from build123d import *

# Parameters (mm, degrees)
SKETCH1_R                             = 7.9375
BOSS_EXTRUDE1_DEPTH                   = 53.467
F_29_0_136_DIAMETER_HOLE1_D           = 3.4544
F_29_0_136_DIAMETER_HOLE1_CSINK_D     = 4.7244
F_29_0_136_DIAMETER_HOLE1_CSINK_ANGLE = 45
F_15_0_18_DIAMETER_HOLE1_D            = 4.572
F_53_0_0595_DIAMETER_HOLE1_D          = 1.5113
F_3_8_0_375_DIAMETER_HOLE1_D          = 9.525
F_3_8_0_375_DIAMETER_HOLE1_DEPTH      = 50.8
F_3_8_0_375_DIAMETER_HOLE1_TIP        = 2.861598698
F_39_0_0995_DIAMETER_HOLE1_D          = 2.54


with BuildPart() as part:
    # Sketch1 → Boss-Extrude1 (new body)
    with BuildSketch(Plane(origin=(0, 0, 0), x_dir=(1, 0, 0), z_dir=(0, 1, 0))):
        with Locations(Location((0, 0, 0), (0, 0, 270))):
            Circle(SKETCH1_R)
    extrude(amount=BOSS_EXTRUDE1_DEPTH)

    # #29 (0.136) Diameter Hole1 (through all)
    with Locations(Plane.XY.offset(7.9375)):
        with Locations((0, 49.022)):
            CounterSinkHole(F_29_0_136_DIAMETER_HOLE1_D / 2, F_29_0_136_DIAMETER_HOLE1_CSINK_D / 2, counter_sink_angle=F_29_0_136_DIAMETER_HOLE1_CSINK_ANGLE)

    # #15 (0.18) Diameter Hole1 (through all)
    with Locations(Plane.XY.offset(7.9375)):
        with Locations((0, 40.64)):
            Hole(F_15_0_18_DIAMETER_HOLE1_D / 2)

    # #53 (0.0595) Diameter Hole1 (through all)
    with Locations(Plane.XY.offset(7.9375)):
        with Locations((0, 32.639)):
            Hole(F_53_0_0595_DIAMETER_HOLE1_D / 2)

    # 3/8 (0.375) Diameter Hole1
    with Locations(Plane(origin=(0, 53.467, 0), x_dir=(1, 0, 0), z_dir=(0, 1, 0))):
        with Locations((0, 0)):
            Hole(F_3_8_0_375_DIAMETER_HOLE1_D / 2, depth=F_3_8_0_375_DIAMETER_HOLE1_DEPTH)
            with Locations((0, 0, -(F_3_8_0_375_DIAMETER_HOLE1_DEPTH + F_3_8_0_375_DIAMETER_HOLE1_TIP / 2))):  # 118° drill point
                Cone(0, F_3_8_0_375_DIAMETER_HOLE1_D / 2, F_3_8_0_375_DIAMETER_HOLE1_TIP, mode=Mode.SUBTRACT)

    # #39 (0.0995) Diameter Hole1 (through all)
    with Locations(Plane(origin=(0, 0, 0), x_dir=(-1, 0, 0), z_dir=(0, -1, 0))):
        with Locations((0, 0)):
            Hole(F_39_0_0995_DIAMETER_HOLE1_D / 2)


solid = part.part
Geometry: final body of the model. Coordinates: model frame, mm. A direction names the side the tool comes from. Give positions to 0.01 mm unless a question says otherwise; leave off trailing zeros. Write each loop counter-clockwise with the first axis right and the second up, starting at its lowest first coordinate (ties: lowest second). Pieces come first, ordered by that corner, then holes. Notation, with made-up numbers: (10.25, -29) - (51.25, -29) arc R13 cw to (51.25, -21) - close; hole circle Ø6 at (-37, 88.5). An arc over 180 degrees is marked (long way). Return JSON: item names as keys, results as strings. Group by question number.
1) Section B-B on y = 41.5. Return the cut outline in (x, z) (1 decimal), plus the area to 3 significant figures.
2) First-contact query: P1, Ø5, axis at x = -5, y = 12.5, coming from the +Z side; P2, Ø2.5, axis at x = 0, y = 40.64, coming from the -Z side; P3, Ø4.5, axis at x = 0, y = 49.022, coming from the +Z side; P4, Ø4, axis at x = 0, y = 49.022, coming from the +Z side. Flat tips, straight axial feed; report the tip coordinate or a pass-through.
3) Set-up query: faces 1 (the cylindrical face through (1.37, 47.97, -6.21)), 2 (the cylindrical face through (-4.543, 27.711, -1.431)). Return all of +Z, -Z, +X, -X, +Y, -Y with unobstructed straight access to the full face (end or side cutting, diameter ignored); none if empty.
4) Line query: line 1 (Y direction, x = 0, z = -6.05); line 2 (Z direction, x = 0, y = 0.45); line 3 (Z direction, x = 0, y = 15). Output: solid intervals per line, ascending.
5) Section D-D on z = 5.5. Return the cut outline in (x, y), plus the area to 3 significant figures.
6) Section A-A on z = 0. Return the cut outline in (x, y).
7) Section C-C on x = 0. State how many separate pieces and enclosed holes the cut face has, plus the area to 3 significant figures.
8) Mould query, pull axis Z, two halves, no side actions, for faces 3 (the flat face through (-5, 53.467, 0)), 4 (the conical face through (1.45, 47.91, 6.65)), 5 (the cylindrical face through (-0.17, 0.29, -1.26)). Classes: released by +Z, released by -Z, zero draft, split by the parting line, or undercut.
Filled in:
{
 "1": {"outline": "(-2.1, -7.6) - (-2.1, -4.3) arc R4.8 cw to (-2.1, 4.3) - (-2.1, 7.6) arc R7.9 ccw to start; (2.1, -7.6) arc R7.9 ccw to (2.1, 7.6) - (2.1, 4.3) arc R4.8 cw to (2.1, -4.3) - close", "area": "99.2 mm^2"},
 "2": {"P1": "stops at z = 7.53", "P2": "passes through", "P3": "stops at z = 7.67", "P4": "stops at z = 7.06"},
 "3": {"face 1": "+Z, -Z", "face 2": "+Y"},
 "4": {"line 1": "y = 0 to 31.88, 33.39 to 38.35, 42.93 to 47.29, 50.75 to 53.47", "line 2": "z = -7.94 to -1.27, 1.27 to 7.94", "line 3": "z = -7.94 to -4.76, 4.76 to 7.94"},
 "5": {"outline": "(-5.72, 0) - (5.72, 0) - (5.72, 53.47) - (-5.72, 53.47) - close; hole circle Ø4.57 at (0, 40.64); hole circle Ø3.45 at (0, 49.02); hole circle Ø1.51 at (0, 32.64)", "area": "584 mm^2"},
 "6": {"outline": "(-7.94, 0) - (-1.27, 0) - (-1.27, 0.57) - (-4.76, 2.67) - (-4.76, 53.47) - (-7.94, 53.47) - close; (1.27, 0) - (7.94, 0) - (7.94, 53.47) - (4.76, 53.47) - (4.76, 2.67) - (1.27, 0.57) - close"},
 "7": {"separate pieces": "8", "enclosed holes": "0", "area": "289 mm^2"},
 "8": {"face 3": "zero draft", "face 4": "released by +Z", "face 5": "undercut"}
}
